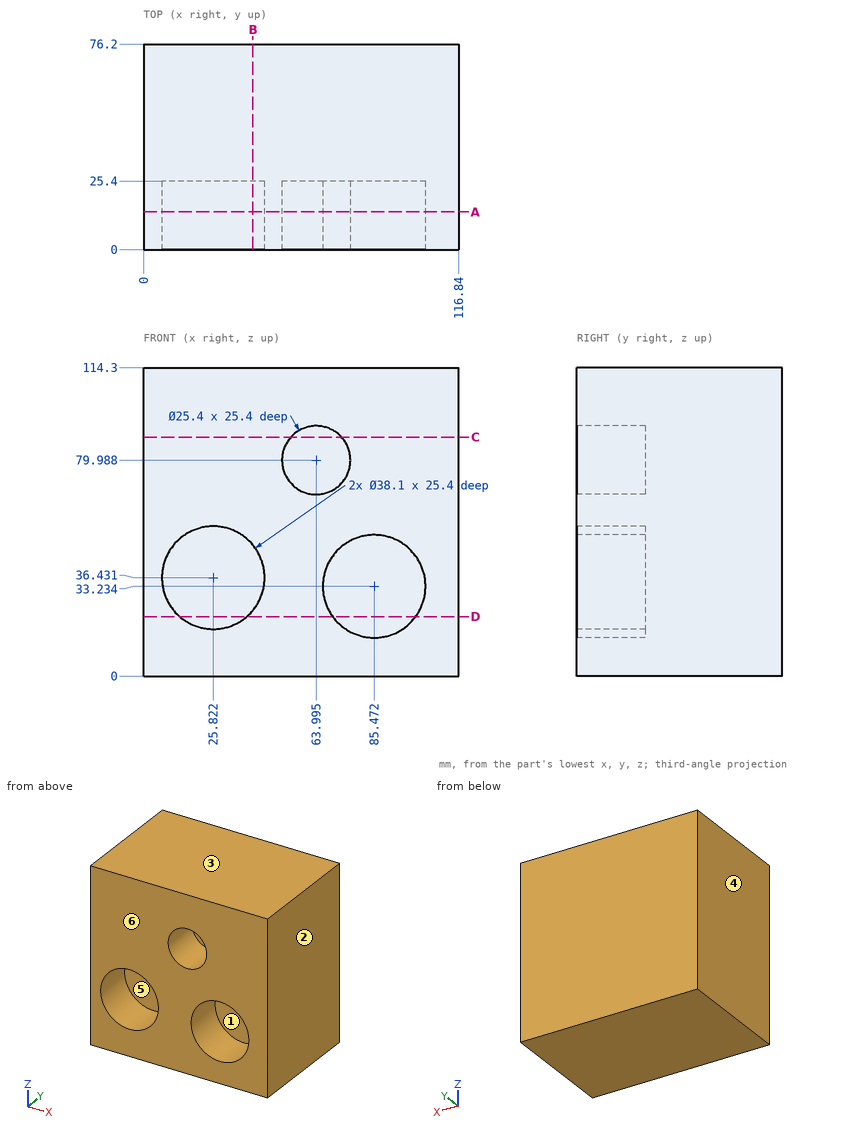
Input: dimensioned drawing with shaded views. Units: mm. Origin: part minimum x, y, z. A direction names the side the tool comes from. Round coordinates to 2 decimals unless told otherwise and drop trailing zeros. Order: outer loops, then holes, each group sorted by start corner. A loop starts at its lowest first (then second) coordinate and runs counter-clockwise, first axis right, second up.
1. Cut plane C-C, the plane z = 88.5. Output: boundary loops of the cut face in (x, y), then the cut area to 3 significant figures.
The answers:
outline: (0, 0) - (54.57, 0) - (54.57, 25.4) - (73.42, 25.4) - (73.42, 0) - (116.84, 0) - (116.84, 76.2) - (0, 76.2) - close
area: 8,420 mm2
2. Set-up query: the marked faces 5 and 6. Return all of +Z, -Z, +X, -X, +Y, -Y with unobstructed straight access to the full face (end or side cutting, diameter ignored); none if empty.
The answers:
face 5: -Y
face 6: +Z, -Z, +X, -X, -Y
3. Mould query, pull axis X, two halves, no side actions, for the marked faces 1, 2, 3 and 4. Classes: released by +X, released by -X, zero draft, split by the parting line, or undercut.
The answers:
face 1: undercut
face 2: released by +X
face 3: zero draft
face 4: released by -X
4. Cut plane A-A, the plane y = 14. State how many separate pieces and enclosed holes the cut face has, then the cut area to 3 significant figures.
The answers:
separate pieces: 1
enclosed holes: 3
area: 10,600 mm2
5. Pin query (flat end, axial travel): P1, Ø12.5, axis at x = 66.5, z = 77, coming from the -Y side. Return the tip coordinate at first contact, or that it passes through.
The answers:
P1: stops at y = 25.4
6. Cut plane B-B, the plane x = 40.5. Output: boundary loops of the cut face in (y, z).
The answers:
outline: (0, 0) - (76.2, 0) - (76.2, 114.3) - (0, 114.3) - (0, 48.57) - (25.4, 48.57) - (25.4, 24.29) - (0, 24.29) - close
7. Cut plane D-D, the plane z = 22. Output: boundary loops of the cut face in (x, y).
The answers:
outline: (0, 0) - (13.39, 0) - (13.39, 25.4) - (38.26, 25.4) - (38.26, 0) - (70.09, 0) - (70.09, 25.4) - (100.86, 25.4) - (100.86, 0) - (116.84, 0) - (116.84, 76.2) - (0, 76.2) - close
8. Material intervals for line 1 (Y direction, x = 35, z = 37.5); line 2 (X direction, y = 17.5, z = 48.5) (1 decimal); line 3 (Z direction, x = 11, y = 22) (1 decimal), sorted ascending.
The answers:
line 1: y = 25.4 to 76.2
line 2: x = 0 to 11.1, 40.6 to 74.1, 96.9 to 116.8
line 3: z = 0 to 24.5, 48.4 to 114.3
